Geometry check sheet. Reference: the model listing, model coordinates, mm. Face numbers are marked on the shaded views. A direction names the side the tool comes from. Give positions to 0.01 mm unless a question says otherwise; leave off trailing zeros. Write each loop counter-clockwise with the first axis right and the second up, starting at its lowest first coordinate (ties: lowest second). Pieces come first, ordered by that corner, then holes. Notation, with made-up numbers: (35, 0) - (86, 0) arc R13 cw to (86, 21) - close; hole circle Ø7 at (-0.5, 42). An arc over 180 degrees is marked (long way). One line per question, with ' | ' between items. Start each with the question number.
Q1. Section check A-A on z = -84. Record the boundary of the cut face in (x, y), and give its area (3 significant figures).
Q2. Set-up check for the marked faces 5, 6, 7, 8 and 9: record each of +Z, -Z, +X, -X, +Y, -Y from which the full face is reachable in a straight line by a thin tool's end or side.
Q3. Section check C-C on y = 6.5. Record the boundary of the cut face in (x, z).
Q4. Thickness scan on L1, parallel to X at y = 20, z = -80; L2, parallel to Z at x = 62, y = 31; L3, parallel to Z at x = 63, y = 6. Record the ranges inside material, lowest first. Write a range as [from, to].
Q5. Release check for a two-part mould opening along Z. For the marked faces 1, 2, 3 and 4 record: +Z half, -Z half, draft (parallel to the pull), parting line (faces both ways), or undercut.
Q6. Section check B-B on x = 89.5. Record the boundary of the cut face in (y, z), and give its area (3 significant figures).
Q7. Section check D-D on y = 45.5. Record the boundary of the cut face in (x, z), and give its area (3 significant figures).
Q8. Gauge pin test, flat ends, axial feed: P1, Ø5, axis at y = 1, z = -45, coming from the -X side; P2, Ø5, axis at x = 70.5, y = 32.5, coming from the -Z side; P3, Ø6, axis at x = 71.5, z = -28, coming from the +Y side. Record the tip position at first contact, or that the pin passes through.
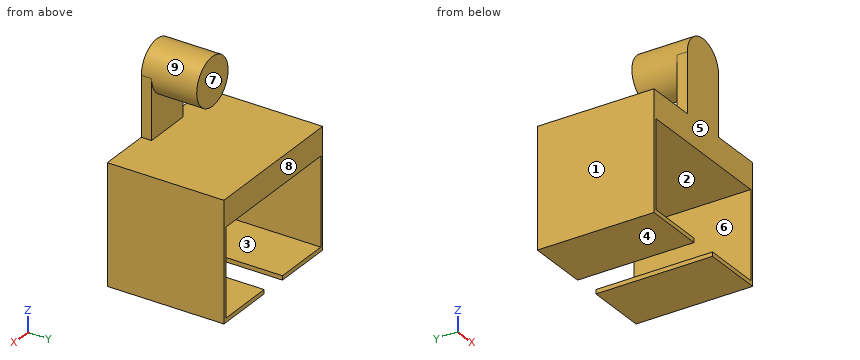
```python
from build123d import *

# Parameters (mm, degrees)
BOSS_EXTRUDE1_DEPTH = 50.8
SKETCH3_W           = 20.832647018
SKETCH3_H           = 4.473256697
BOSS_EXTRUDE2_DEPTH = 25.908
SKETCH5_R           = 10.416323509
BOSS_EXTRUDE3_DEPTH = 24.13


with BuildPart() as part:
    # Sketch2 → Boss-Extrude1 (new body)
    with BuildSketch(Plane(origin=(0, 0, 0), x_dir=(1, 0, 0), z_dir=(0, 1, 0))):
        Polygon((66.696577012, 107.786627361), (66.696577012, 105.952916401), (41.286417012, 105.952916401), (41.286417012, 67.871966401), (104.329217012, 67.871966401), (104.329217012, 105.952916401), (78.919057012, 105.952916401), (78.919057012, 107.786627361), (105.573817012, 107.786627361), (105.573817012, 56.048909831), (40.041817012, 56.048909831), (40.041817012, 107.786627361), align=None)
    extrude(amount=BOSS_EXTRUDE1_DEPTH)

    # Sketch3 → Boss-Extrude2 (add)
    with BuildSketch(Plane.XY.offset(-56.048909831)):
        with Locations((72.594457012, 2.236628349)):
            Rectangle(SKETCH3_W, SKETCH3_H)
    extrude(amount=BOSS_EXTRUDE2_DEPTH)

    # Sketch5 → Boss-Extrude3 (add)
    with BuildSketch(Plane.XZ):
        with Locations(Location((72.594457012, -30.140909831, 0), (0, 0, 270))):
            Circle(SKETCH5_R)
    extrude(amount=-BOSS_EXTRUDE3_DEPTH)


solid = part.part
```
Working result:
1) outline: (40.04, 0) - (41.29, 0) - (41.29, 50.8) - (40.04, 50.8) - close; (104.33, 0) - (105.57, 0) - (105.57, 50.8) - (104.33, 50.8) - close | area: 126 mm2
2) face 5: +Z, -Z, +X, -X, -Y | face 6: +Y, -Y | face 7: +Z, +X, -X, +Y | face 8: +Z, -Z, +X, -X, +Y | face 9: +Y
3) outline: (40.04, -107.79) - (66.7, -107.79) - (66.7, -105.95) - (41.29, -105.95) - (41.29, -67.87) - (104.33, -67.87) - (104.33, -105.95) - (78.92, -105.95) - (78.92, -107.79) - (105.57, -107.79) - (105.57, -56.05) - (40.04, -56.05) - close; circle Ø20.83 at (72.59, -30.14)
4) L1: x = [40.04, 41.29], [104.33, 105.57] | L2: z = [-107.79, -105.95], [-67.87, -56.05] | L3: z = [-107.79, -105.95], [-67.87, -56.05], [-34.2, -26.09]
5) face 1: draft | face 2: undercut | face 3: undercut | face 4: -Z half
6) outline: (0, -107.79) - (50.8, -107.79) - (50.8, -105.95) - (0, -105.95) - close; (0, -67.87) - (50.8, -67.87) - (50.8, -56.05) - (0, -56.05) - close | area: 694 mm2
7) outline: (40.04, -107.79) - (66.7, -107.79) - (66.7, -105.95) - (41.29, -105.95) - (41.29, -67.87) - (104.33, -67.87) - (104.33, -105.95) - (78.92, -105.95) - (78.92, -107.79) - (105.57, -107.79) - (105.57, -56.05) - (40.04, -56.05) - close | area: 967 mm2
8) P1: stops at x = 62.18 | P2: stops at z = -67.87 | P3: stops at y = 24.13
